Source: CAD feature listing. Evaluate the final solid. Frame: model axes, mm. Face numbers are marked on the shaded views. A direction names the side the tool comes from. Coordinates: 2 decimals unless noted, no trailing zeros. Write each loop counter-clockwise with the first axis right and the second up, starting at its lowest first coordinate (ties: lowest second). Pieces come first, ordered by that corner, then holes. Notation, with made-up numbers: M 31.25,-6.75 L 35.25,-6.75 A17 cw 35.25,15.25 Z; hole C 30,80 d3. An arc over 180 degrees is marked long. One line per item, written item: value. Start each with the question number.
Item 1: Ray query, L1, parallel to Z at x = -0.5, y = 9; L2, parallel to X at y = 0.5, z = -20; L3, parallel to Y at x = -4.75, z = -4. Return the intervals inside material, ascending. Write a range as from..to.
Item 2: Cut plane B-B, the plane z = -20. Output: boundary loops of the cut face in (x, y), then the cut area to 3 significant figures.
Item 3: Set-up query: the marked faces 1, 2 and 3. Return all of +Z, -Z, +X, -X, +Y, -Y with unobstructed straight access to the full face (end or side cutting, diameter ignored); none if empty.
Item 4: Pin query (flat end, axial travel): P1, Ø3, axis at y = 4.5, z = -4.5, coming from the -X side (1 decimal); P2, Ø5, axis at x = -0.5, y = 9, coming from the +Z side; P3, Ø3, axis at x = -1.5, y = 5.5, coming from the +Z side. Return the tip coordinate at first contact, or that it passes through.
Item 5: Cut plane C-C, the plane z = 18. Output: boundary loops of the cut face in (x, y).
Item 6: Cut plane D-D, the plane y = 8.75. State how many separate pieces and enclosed holes the cut face has, then the cut area to 3 significant figures.
Item 7: Cut plane A-A, the plane x = 0. Output: boundary loops of the cut face in (y, z).
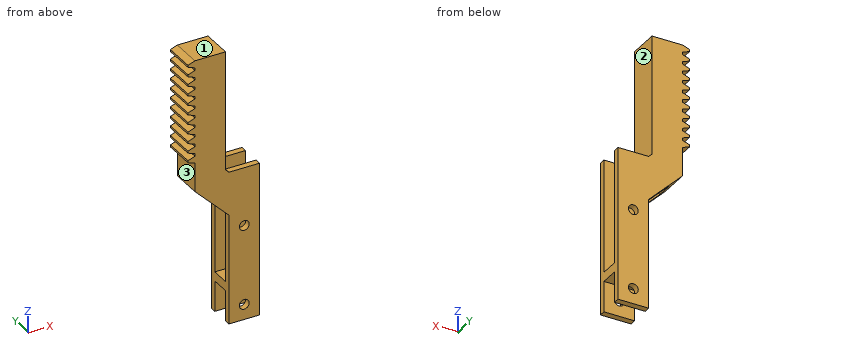
```python
from build123d import *

# Parameters (mm, degrees)
SKETCH_1_W             = 10
SKETCH_1_H             = 50
EXTRUDE_1_DEPTH        = 2
CUT_EXTRUDE_1_REACH    = 27.573
SKETCH_2_R             = 1.6
EXTRUDE_5_DEPTH        = 2
SKETCH_4_W             = 10
SKETCH_4_H             = 3
EXTRUDE_2_DEPTH        = 6
EXTRUDE_START          = 2
SKETCH_5_R             = 1.6
EXTRUDE_3_DEPTH        = 2
EXTRUDE_4_DEPTH        = 10
PATTERN_LINEAR_1_COUNT = 11
PATTERN_LINEAR_1_PITCH = 3.141592654


with BuildPart() as part:
    # 草图1 → 凸台-拉伸1 (new body)
    with BuildSketch(Plane(origin=(0, 0, 0), x_dir=(1, 0, 0), z_dir=(0, 1, 0))):
        Rectangle(SKETCH_1_W, SKETCH_1_H)
    extrude(amount=EXTRUDE_1_DEPTH)

    # 草图2 → 切除-拉伸1 (cut, up to next)
    with BuildSketch(Plane(origin=(0, 2, 0), x_dir=(1, 0, 0), z_dir=(0, 1, 0)), mode=Mode.PRIVATE) as cut_extrude_1_sk1:
        with Locations(Location((0, 20, 0), (0, 0, 270))):
            Circle(SKETCH_2_R)
    cut_extrude_1_tool1 = extrude(cut_extrude_1_sk1.sketch, amount=-CUT_EXTRUDE_1_REACH, mode=Mode.PRIVATE) & part.part
    # 草图2 → 切除-拉伸1 (cut, up to next)
    with BuildSketch(Plane(origin=(0, 2, 0), x_dir=(1, 0, 0), z_dir=(0, 1, 0)), mode=Mode.PRIVATE) as cut_extrude_1_sk2:
        with Locations(Location((0, -5.98075, 0), (0, 0, 270))):
            Circle(SKETCH_2_R)
    cut_extrude_1_tool2 = extrude(cut_extrude_1_sk2.sketch, amount=-CUT_EXTRUDE_1_REACH, mode=Mode.PRIVATE) & part.part
    add(cut_extrude_1_tool1.solids().sort_by_distance((0, 2, -20))[0], mode=Mode.SUBTRACT)
    add(cut_extrude_1_tool2.solids().sort_by_distance((0, 2, 5.98075))[0], mode=Mode.SUBTRACT)

    # 草图8 → 凸台-拉伸5 (add)
    with BuildSketch(Plane(origin=(0, 2, 0), x_dir=(1, 0, 0), z_dir=(0, 1, 0))):
        Polygon((-5, -25), (-6.07, -26.07), (-6.07, -65), (-16.07, -65), (-16.07, -21.927864376), (-5, -10.857864376), align=None)
    extrude(amount=-EXTRUDE_5_DEPTH)

    # 草图4 → 凸台-拉伸2 (add)
    with BuildSketch(Plane(origin=(0, 2, 0), x_dir=(1, 0, 0), z_dir=(0, 1, 0))):
        with Locations((0, 13.5)):
            Rectangle(SKETCH_4_W, SKETCH_4_H)
        Polygon((-6.07, -26.07), (-13.141067812, -18.998932188), (-16.07, -21.927864376), (-16.07, -65), (-6.07, -65), align=None)
    extrude(amount=EXTRUDE_2_DEPTH)

    # 草图5 → 凸台-拉伸3 (add)
    with BuildSketch(Plane(origin=(0, 8, 0), x_dir=(1, 0, 0), z_dir=(0, 1, 0)).offset(EXTRUDE_START)):
        Polygon((-5, 25), (-5, -10.857864376), (-16.07, -21.927864376), (-16.07, -65), (-6.07, -65), (-6.07, -26.07), (-5, -25), (5, -25), (5, 25), align=None)
        with Locations(Location((0, -5.98075, 0), (0, 0, 270))):
            Circle(SKETCH_5_R, mode=Mode.SUBTRACT)
        with Locations(Location((0, 20, 0), (0, 0, 270))):
            Circle(SKETCH_5_R, mode=Mode.SUBTRACT)
    extrude(amount=-EXTRUDE_3_DEPTH)

    # 草图7 → 凸台-拉伸4 (add)
    with BuildSketch(Plane(origin=(0, 10, 0), x_dir=(1, 0, 0), z_dir=(0, 1, 0))):
        Polygon((-16.07, -65), (-18.32, -64.181066973), (-18.32, -63.520196234), (-16.07, -62.701263206), align=None)
    extrude_4 = extrude(amount=-EXTRUDE_4_DEPTH)

    # 阵列(线性)1: 凸台-拉伸4 ×11
    with Locations(*[(0, 0, -i * PATTERN_LINEAR_1_PITCH) for i in range(1, PATTERN_LINEAR_1_COUNT)]):
        add(extrude_4)


solid = part.part
```
From the geometry:
1. L1: z = -25..-21.52, -18.48..4.46, 7.5..25
1. L2: x = -5..-1.6, 1.6..5
1. L3: y = 0..2, 8..10
2. outline: M -5,0 L -1.6,0 L -1.6,2 L -5,2 Z; M -5,8 L -1.6,8 L -1.6,10 L -5,10 Z; M 1.6,0 L 5,0 L 5,2 L 1.6,2 Z; M 1.6,8 L 5,8 L 5,10 L 1.6,10 Z
2. area: 27.2 mm²
3. face 1: +Z, +X, -X, +Y, -Y
3. face 2: +Z, +X, +Y, -Y
3. face 3: -Z, -X, +Y, -Y
4. P1: passes through
4. P2: stops at z = 25
4. P3: stops at z = -12
5. outline: M -12.14,0 L 5,0 L 5,2 L -12.14,2 Z; M -12.14,8 L 5,8 L 5,10 L -12.14,10 Z
6. separate pieces: 1
6. enclosed holes: 2
6. area: 1,020 mm²
7. outline: M 0,-25 L 2,-25 L 2,-21.6 L 0,-21.6 Z; M 0,-18.4 L 2,-18.4 L 2,-15 L 8,-15 L 8,-18.4 L 10,-18.4 L 10,4.38 L 8,4.38 L 8,-12 L 2,-12 L 2,4.38 L 0,4.38 Z; M 0,7.58 L 2,7.58 L 2,25 L 0,25 Z; M 8,-25 L 10,-25 L 10,-21.6 L 8,-21.6 Z; M 8,7.58 L 10,7.58 L 10,25 L 8,25 Z
